```python
from build123d import *

# Parameters (mm, degrees)
BOSS_EXTRUDE1_DEPTH = 30
BOSS_EXTRUDE2_DEPTH = 5
BOSS_EXTRUDE3_DEPTH = 5
SKETCH5_R           = 2.25
CUT_EXTRUDE1_DEPTH  = 12.5


with BuildPart() as part:
    # Sketch2 → Boss-Extrude1 (new body)
    with BuildSketch(Plane.XY):
        with BuildLine():
            Line((0, 0), (0, 12.5))
            Line((0, 12.5), (70, 12.5))
            Line((70, 12.5), (70, 0))
            Line((70, 0), (60, 0))
            ThreePointArc((60, 0), (52.5, 7.5), (45, 0))
            Line((45, 0), (25, 0))
            ThreePointArc((25, 0), (17.5, 7.5), (10, 0))
            Line((10, 0), (0, 0))
        make_face()
    extrude(amount=BOSS_EXTRUDE1_DEPTH)

    # Sketch3 → Boss-Extrude2 (add)
    with BuildSketch(Plane.XY.offset(30)):
        with BuildLine():
            Line((17.5, 12.5), (52.5, 12.5))
            ThreePointArc((52.5, 12.5), (61.338834765, 8.838834765), (65, 0))
            Line((65, 0), (60, 0))
            ThreePointArc((60, 0), (52.5, 7.5), (45, 0))
            Line((45, 0), (25, 0))
            ThreePointArc((25, 0), (17.5, 7.5), (10, 0))
            Line((10, 0), (5, 0))
            ThreePointArc((5, 0), (8.661165235, 8.838834765), (17.5, 12.5))
        make_face()
    extrude(amount=BOSS_EXTRUDE2_DEPTH)

    # Sketch4 → Boss-Extrude3 (add)
    with BuildSketch(Plane(origin=(0, 0, 0), x_dir=(-1, 0, 0), z_dir=(0, 0, -1))):
        with BuildLine():
            Line((-65, 0), (-60, 0))
            ThreePointArc((-60, 0), (-52.5, 7.5), (-45, 0))
            Line((-45, 0), (-25, 0))
            ThreePointArc((-25, 0), (-17.5, 7.5), (-10, 0))
            Line((-10, 0), (-5, 0))
            ThreePointArc((-5, 0), (-8.661165235, 8.838834765), (-17.5, 12.5))
            Line((-17.5, 12.5), (-52.5, 12.5))
            ThreePointArc((-52.5, 12.5), (-61.338834765, 8.838834765), (-65, 0))
        make_face()
    extrude(amount=BOSS_EXTRUDE3_DEPTH)

    # Sketch5 → Cut-Extrude1 (cut)
    with BuildSketch(Plane(origin=(0, 12.5, 0), x_dir=(1, 0, 0), z_dir=(0, 1, 0))):
        with Locations((35, 0)):
            Circle(SKETCH5_R)
        with Locations((35, -30)):
            Circle(SKETCH5_R)
        with Locations((65, -7.5)):
            Circle(SKETCH5_R)
        with Locations((65, -22.5)):
            Circle(SKETCH5_R)
        with Locations((5, -22.5)):
            Circle(SKETCH5_R)
        with Locations((5, -7.5)):
            Circle(SKETCH5_R)
    extrude(amount=-CUT_EXTRUDE1_DEPTH, mode=Mode.SUBTRACT)


solid = part.part
```
The listing builds one solid part. Answer for the finished solid, in the listing's coordinates (mm). A direction names the side the tool comes from. Round coordinates to 2 decimals unless told otherwise and drop trailing zeros. Order: outer loops, then holes, each group sorted by start corner. A loop starts at its lowest first (then second) coordinate and runs counter-clockwise, first axis right, second up. Notation, with made-up numbers: (-32.5, -2) -> (-14.5, -2) arc R18 cw to (-14.5, 10) -> close; hole circle Ø2 at (-25, -7). An arc over 180 degrees is marked (long way). Answer as CSV lines item,"result". Start each with the question number.
(1) Find the intervals of material crossed by probe 1 along Z at (x, y) = (65, 3.75); probe 2 along X at (y, z) = (0.5, 10); probe 3 along Z at (x, y) = (35, 8.25), in increasing order. Write a range as from..to.
(2) The part is cut by section A-A (y = 5.25). Count the separate pieces of the cut face and the enclosed holes in it, then the cut area to 3 significant figures.
(3) A tool of negligible diameter and unlimited length cuts with its end or side. For faces 1 (the face through (61.241, 8.935, -2.465)), 2 (the face through (8.565, 8.741, 32.465)), 3 (the face through (5, 8, 0)), 4 (the face through (61.241, 8.935, 32.465)), from which of +Z, -Z, +X, -X, +Y, -Y can it reach the whole face along a straight path? Write none if from no direction.
(4) For a pull along Z with two mould halves and no side action, classify faces 5 (the face through (37.08, 6.34, 30.86)), 6 (the face through (4.512, 6.338, 24.696)), 7 (the face through (65, 8, 0)), 8 (the face through (52.66, 7.5, 15.28)) as +Z half, -Z half, draft (parallel to the pull), parting line (faces both ways), or undercut.
(5) The part is cut by section D-D (z = 19). Determine the outline of the cut face in (x, y).
(6) A flat-ended cylindrical pin translates along its axis: pin 1 Ø3.5 at (x, z) = (35, 0) entering from -Y. Find the tip coordinate at first contact, or state that the pin passes through.
(7) The part is cut by section B-B (z = 7.5). Determine the outline of the cut face in (x, y).
(8) The part is cut by section C-C (x = 35). Determine the outline of the cut face in (y, z).
Evaluation:
1,probe 1,"0..5.25, 9.75..20.25, 24.75..30"
1,probe 2,"0..10.02, 24.98..45.02, 59.98..70"
1,probe 3,"-5..-2.25, 2.25..27.75, 32.25..35"
2,separate pieces,"3"
2,enclosed holes,"6"
2,area,"1,720 mm²"
3,face 1,"-Z, +X, +Y"
3,face 2,"+Z, -X, +Y"
3,face 3,"-Z, -X, +Y"
3,face 4,"+Z, +X, +Y"
4,face 5,"undercut"
4,face 6,"undercut"
4,face 7,"-Z half"
4,face 8,"draft"
5,outline,"(0, 0) -> (10, 0) arc R7.5 cw to (25, 0) -> (45, 0) arc R7.5 cw to (60, 0) -> (70, 0) -> (70, 12.5) -> (0, 12.5) -> close"
6,pin 1,"through"
7,outline,"(0, 0) -> (2.75, 0) -> (2.75, 12.5) -> (0, 12.5) -> close; (7.25, 0) -> (10, 0) arc R7.5 cw to (25, 0) -> (45, 0) arc R7.5 cw to (60, 0) -> (62.75, 0) -> (62.75, 12.5) -> (7.25, 12.5) -> close; (67.25, 0) -> (70, 0) -> (70, 12.5) -> (67.25, 12.5) -> close"
8,outline,"(0, -5) -> (12.5, -5) -> (12.5, -2.25) -> (0, -2.25) -> close; (0, 2.25) -> (12.5, 2.25) -> (12.5, 27.75) -> (0, 27.75) -> close; (0, 32.25) -> (12.5, 32.25) -> (12.5, 35) -> (0, 35) -> close"
